Geometry: see drawing. Coordinates: mm, zero at the bounding-box minimum. Round coordinates to 2 decimals unless told otherwise and drop trailing zeros. Write each loop counter-clockwise with the first axis right and the second up, starting at its lowest first coordinate (ties: lowest second). Pieces come first, ordered by that corner, then holes.
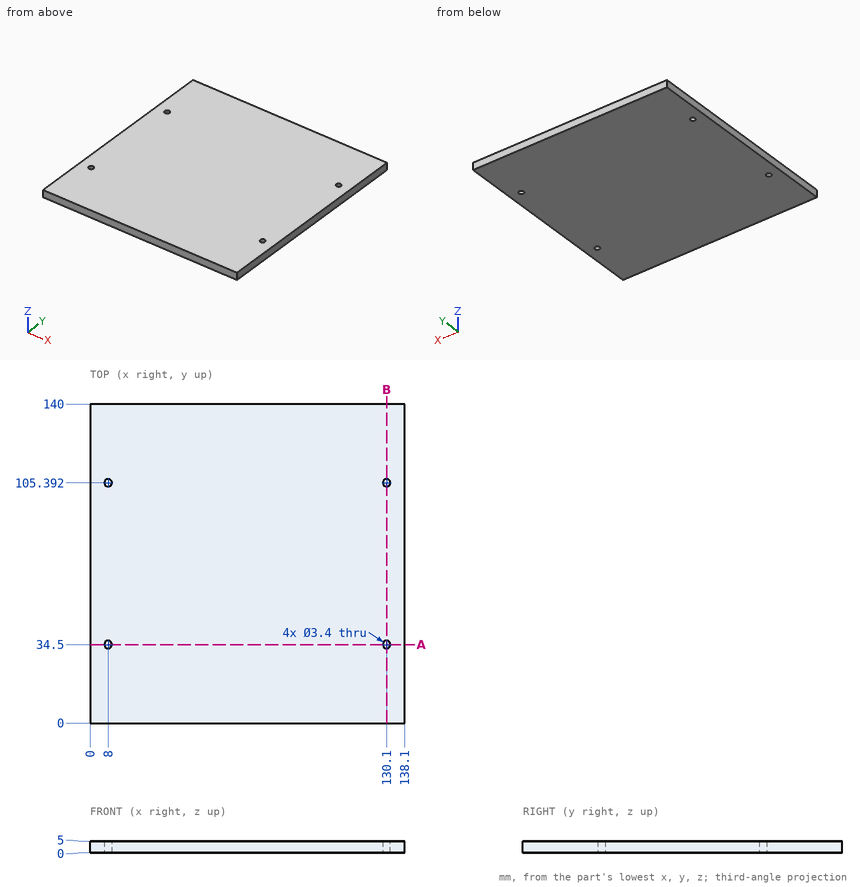
Q1. Line query: line 1 (Y direction, x = 130.1, z = 1.75); line 2 (X direction, y = 104, z = 2.05). Output: solid intervals per line, ascending.
Q2. Section query B-B, the plane x = 130.1. Output: boundary loops of the cut face in (y, z), and give its area (3 significant figures).
Q3. Section query A-A, the plane y = 34.5. Output: boundary loops of the cut face in (x, z).
Q4. Pin query (flat end, axial travel): P1, Ø2, axis at x = 8, y = 105.39, coming from the -Z side. Return the tip coordinate at first contact, or that it passes through.
Filled in:
1. line 1: y = 0 to 32.8, 36.2 to 103.69, 107.09 to 140
1. line 2: x = 0 to 7.02, 8.98 to 129.12, 131.08 to 138.1
2. outline: (0, 0) - (32.8, 0) - (32.8, 5) - (0, 5) - close; (36.2, 0) - (103.69, 0) - (103.69, 5) - (36.2, 5) - close; (107.09, 0) - (140, 0) - (140, 5) - (107.09, 5) - close
2. area: 666 mm2
3. outline: (0, 0) - (6.3, 0) - (6.3, 5) - (0, 5) - close; (9.7, 0) - (128.4, 0) - (128.4, 5) - (9.7, 5) - close; (131.8, 0) - (138.1, 0) - (138.1, 5) - (131.8, 5) - close
4. P1: passes through
